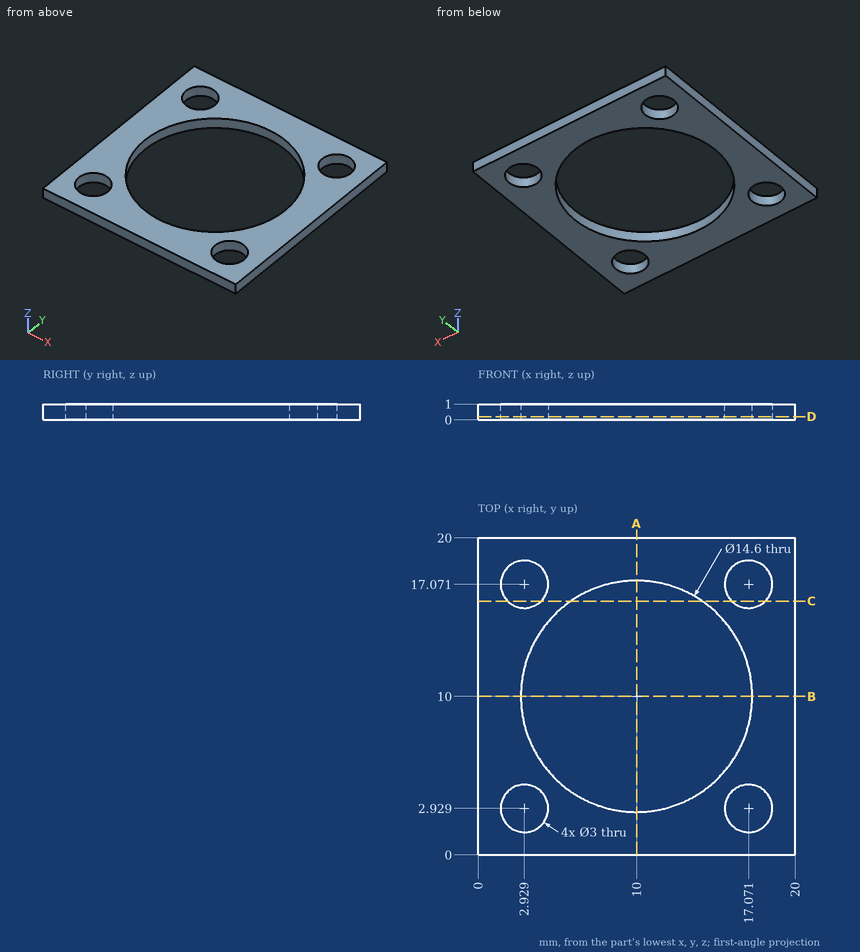
Input: dimensioned drawing with shaded views. Units: mm. Origin: part minimum x, y, z. Round coordinates to 2 decimals unless told otherwise and drop trailing zeros. Order: outer loops, then holes, each group sorted by start corner. A loop starts at its lowest first (then second) coordinate and runs counter-clockwise, first axis right, second up. Notation, with made-up numbers: (77, -9.5) - (115, -9.5) arc R19 ccw to (115, 2.5) - close; hole circle Ø5 at (47.25, 8.5). An arc over 180 degrees is marked (long way). Write item = value, one per line. Start each with the question number.
Q1. Cut plane A-A on x = 10. Return the cut outline in (y, z), and give its area (3 significant figures).
Q2. Ray query, line 1 (Y direction, x = 10, z = 0.7); line 2 (X direction, y = 2.25, z = 0.15); line 3 (X direction, y = 18, z = 0.9). Return the intervals inside material, ascending. Write a range as from..to.
Q3. Cut plane D-D on z = 0.2. Return the cut outline in (x, y), and give its area (3 significant figures).
Q4. Cut plane C-C on y = 16. Return the cut outline in (x, z).
Outcome:
q1.outline = (0, 0) - (2.7, 0) - (2.7, 1) - (0, 1) - close; (17.3, 0) - (20, 0) - (20, 1) - (17.3, 1) - close
q1.area = 5.40 mm^2
q2.line_1 = 0..2.7, 17.3..20
q2.line_2 = 0..1.59, 4.27..15.73, 18.41..20
q2.line_3 = 0..1.75, 4.11..15.89, 18.25..20
q3.outline = (0, 0) - (20, 0) - (20, 20) - (0, 20) - close; hole circle Ø3 at (2.93, 2.93); hole circle Ø3 at (2.93, 17.07); hole circle Ø14.6 at (10, 10); hole circle Ø3 at (17.07, 2.93); hole circle Ø3 at (17.07, 17.07)
q3.area = 204 mm^2
q4.outline = (0, 0) - (1.88, 0) - (1.88, 1) - (0, 1) - close; (3.98, 0) - (5.84, 0) - (5.84, 1) - (3.98, 1) - close; (14.16, 0) - (16.02, 0) - (16.02, 1) - (14.16, 1) - close; (18.12, 0) - (20, 0) - (20, 1) - (18.12, 1) - close
